Geometry: final body of the model. Coordinates: model frame, mm. Face numbers are marked on the shaded views. A direction names the side the tool comes from. Round coordinates to 2 decimals unless told otherwise and drop trailing zeros. Write each loop counter-clockwise with the first axis right and the second up, starting at its lowest first coordinate (ties: lowest second). Pieces come first, ordered by that corner, then holes. Notation, with made-up numbers: M 38.5,78 L 86.5,78 A26 ccw 86.5,92 Z; hole C 34,44.25 d6. An arc over 180 degrees is marked long. Answer as CSV lines item,"result". Start each with the question number.
Q1. Section query B-B on y = 0. Give the number of separate pieces and of enclosed holes in the cut face, and give its area (3 significant figures).
Q2. Mould query, pull axis Z, two halves, no side actions, for the marked faces 4, 5 and 6. Classes: pulls with the +Z half, pulls with the -Z half, needs draft (parallel to the pull), parting line crosses it, or undercut.
Q3. Reachability of the marked faces 1, 2 and 3 from +Z, -Z, +X, -X, +Y, -Y: full face, straight path, thin tool, end or side. Return the list, or none.
Q4. Ray query, probe 1 along Y at (x, z) = (-12.5, -1); probe 2 along Y at (x, z) = (7.5, -8.6); probe 3 along X at (y, z) = (5.25, 6.25). Return the intervals inside material, ascending.
Q5. Section query C-C on x = -17. Output: boundary loops of the cut face in (y, z).
Q6. Section query A-A on x = 7.5. Output: boundary loops of the cut face in (y, z).
Q7. First-contact query: pin 1 (2.5 mm diameter, centred on x = -12.5, y = -8.75, fed in from -Z); pin 2 (6 mm diameter, centred on x = 19, z = -2.5, fed in from +Y); pin 3 (1 mm diameter, centred on y = -8.5, z = -5.5, fed in from +X); pin 4 (1.5 mm diameter, centred on x = 23, z = -0.5, fed in from -Y). Flat tips, straight axial feed; report the tip coordinate or a pass-through.
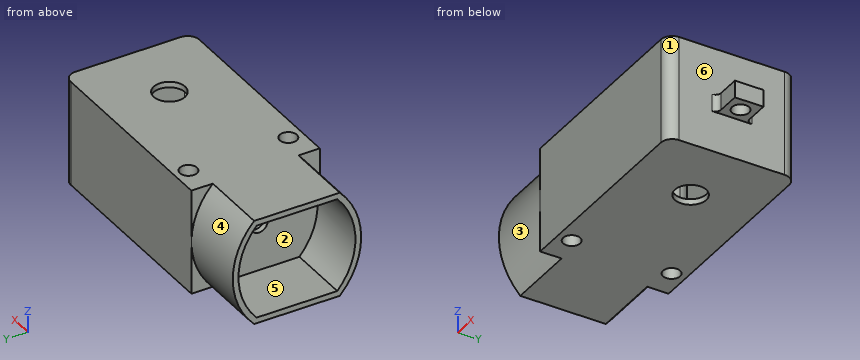
```python
from build123d import *

# Parameters (mm, degrees)
SKETCH1_R                = 1.5
BOSS_EXTRUDE1_DEPTH      = 9.22
BOSS_EXTRUDE2_DEPTH      = 12
SHELL1_START             = -10
SHELL1_OUTLINE_W         = 20.5
SHELL1_OUTLINE_H         = 16.44
SHELL1_DEPTH             = 27.5
SHELL1_START_2           = -29.5
SHELL1_2_DEPTH           = 14.5
SHELL1_START_3           = -16.5
SHELL1_3_DEPTH           = 1.5
SHELL1_START_4           = -8.22
SHELL1_4_DEPTH           = 16.44
SKETCH3_R                = 1.5
BOSS_EXTRUDE3_DEPTH      = 1
BOSS_EXTRUDE4_DEPTH      = 1.5
BOSS_EXTRUDE4_DEPTH_BACK = 1.5
SKETCH6_W                = 5
SKETCH6_H                = 5
SKETCH6_R                = 1.5
SKETCH7_R                = 2.75
CUT_EXTRUDE1_DEPTH       = 37.562906066
FILLET1_R                = 1


with BuildPart() as part:
    # Sketch1 → Boss-Extrude1 (new, symmetric)
    with BuildSketch(Plane.XY):
        with BuildLine():
            Line((17.5, -11.25), (-17.5, -11.25))
            Line((-17.5, -11.25), (-17.5, 11.25))
            Line((-17.5, 11.25), (17.5, 11.25))
            ThreePointArc((17.5, 11.25), (18.914213562, 10.664213562), (19.5, 9.25))
            Line((19.5, 9.25), (19.5, -9.25))
            ThreePointArc((19.5, -9.25), (18.914213562, -10.664213562), (17.5, -11.25))
        make_face()
        with Locations((-12.5, 8.75)):
            Circle(SKETCH1_R, mode=Mode.SUBTRACT)
        with Locations((-12.5, -8.75)):
            Circle(SKETCH1_R, mode=Mode.SUBTRACT)
    extrude(amount=BOSS_EXTRUDE1_DEPTH, both=True)

    # Sketch2 → Boss-Extrude2 (add)
    with BuildSketch(Plane.ZY.offset(17.5)):
        with BuildLine():
            Line((9.22, -7.5), (9.22, 7.5))
            ThreePointArc((9.22, 7.5), (0, 11.25), (-9.22, 7.5))
            Line((-9.22, 7.5), (-9.22, -7.5))
            ThreePointArc((-9.22, -7.5), (0, -11.25), (9.22, -7.5))
        make_face()
    extrude(amount=BOSS_EXTRUDE2_DEPTH)

    # Shell1: read off the stored shape, not the designer's step
    # Shell1 outline → Shell1 (cut)
    with BuildSketch(Plane.YZ.offset(SHELL1_START)):
        Rectangle(SHELL1_OUTLINE_W, SHELL1_OUTLINE_H)
    extrude(amount=SHELL1_DEPTH, mode=Mode.SUBTRACT)

    # Shell1 2 outline → Shell1 2 (cut)
    with BuildSketch(Plane.YZ.offset(SHELL1_START_2)):
        with BuildLine():
            ThreePointArc((7.068411902, -8.22), (10.25, 0), (7.068411902, 8.22))
            Line((7.068411902, 8.22), (-7.068411902, 8.22))
            ThreePointArc((-7.068411902, 8.22), (-10.25, 0), (-7.068411902, -8.22))
            Line((-7.068411902, -8.22), (7.068411902, -8.22))
        make_face()
    extrude(amount=SHELL1_2_DEPTH, mode=Mode.SUBTRACT)

    # Shell1 3 outline → Shell1 3 (cut)
    with BuildSketch(Plane.YZ.offset(SHELL1_START_3)):
        with BuildLine():
            Line((10.25, 0), (10.25, 8.22))
            Line((10.25, 8.22), (7.068411902, 8.22))
            ThreePointArc((7.068411902, 8.22), (9.426855331, 4.407122157), (10.25, 0))
        make_face()
        with BuildLine():
            Line((10.25, -8.22), (10.25, 0))
            ThreePointArc((10.25, 0), (9.426855331, -4.407122157), (7.068411902, -8.22))
            Line((7.068411902, -8.22), (10.25, -8.22))
        make_face()
        with BuildLine():
            ThreePointArc((-10.25, 0), (-9.426855331, 4.407122157), (-7.068411902, 8.22))
            Line((-7.068411902, 8.22), (-10.25, 8.22))
            Line((-10.25, 8.22), (-10.25, 0))
        make_face()
        with BuildLine():
            Line((-10.25, -8.22), (-7.068411902, -8.22))
            ThreePointArc((-7.068411902, -8.22), (-9.426855331, -4.407122157), (-10.25, 0))
            Line((-10.25, 0), (-10.25, -8.22))
        make_face()
    extrude(amount=SHELL1_3_DEPTH, mode=Mode.SUBTRACT)

    # Shell1 4 outline → Shell1 4 (cut)
    with BuildSketch(Plane.XY.offset(SHELL1_START_4)):
        with BuildLine():
            ThreePointArc((-14.5, -10.25), (-14.871708245, -9.540569415), (-15, -8.75))
            Line((-15, -8.75), (-15, -10.25))
            Line((-15, -10.25), (-14.5, -10.25))
        make_face()
        with BuildLine():
            ThreePointArc((-10, 8.75), (-12.499999993, 6.25), (-15, 8.749999987))
            Line((-15, 8.749999987), (-15, -8.75))
            ThreePointArc((-15, -8.75), (-12.5, -6.25), (-10, -8.75))
            Line((-10, -8.75), (-10, 8.75))
        make_face()
        with BuildLine():
            Line((-14.5, 10.25), (-15, 10.25))
            Line((-15, 10.25), (-15, 8.749999987))
            ThreePointArc((-15, 8.749999987), (-14.871708247, 9.540569409), (-14.5, 10.25))
        make_face()
        with BuildLine():
            ThreePointArc((-10.5, 10.25), (-10.128291755, 9.540569415), (-10, 8.75))
            Line((-10, 8.75), (-10, 10.25))
            Line((-10, 10.25), (-10.5, 10.25))
        make_face()
        with BuildLine():
            Line((-10, -10.25), (-10, -8.75))
            ThreePointArc((-10, -8.75), (-10.128291755, -9.540569415), (-10.5, -10.25))
            Line((-10.5, -10.25), (-10, -10.25))
        make_face()
        with BuildLine():
            ThreePointArc((18.5, 9.25), (18.207106781, 9.957106781), (17.5, 10.25))
            Line((17.5, 10.25), (17.5, -10.25))
            ThreePointArc((17.5, -10.25), (18.207106781, -9.957106781), (18.5, -9.25))
            Line((18.5, -9.25), (18.5, 9.25))
        make_face()
    extrude(amount=SHELL1_4_DEPTH, mode=Mode.SUBTRACT)

    # Sketch3 → Boss-Extrude3 (add)
    with BuildSketch(Plane.ZY.offset(17.5)):
        with BuildLine():
            Line((-9.22, 7.5), (-9.22, -7.5))
            ThreePointArc((-9.22, -7.5), (0, -11.25), (9.22, -7.5))
            Line((9.22, -7.5), (9.22, 7.5))
            ThreePointArc((9.22, 7.5), (0, 11.25), (-9.22, 7.5))
        make_face()
        Circle(SKETCH3_R, mode=Mode.SUBTRACT)
    extrude(amount=BOSS_EXTRUDE3_DEPTH)

    # Sketch6 → Boss-Extrude4 (add, two sides: drawn at the far end of the back side and taken through both)
    with BuildSketch(Plane.XY.offset(-0.58).offset(-BOSS_EXTRUDE4_DEPTH_BACK)):
        with Locations((22, 0)):
            Rectangle(SKETCH6_W, SKETCH6_H)
        with Locations((22, 0)):
            Circle(SKETCH6_R, mode=Mode.SUBTRACT)
    extrude(amount=BOSS_EXTRUDE4_DEPTH + BOSS_EXTRUDE4_DEPTH_BACK)

    # Sketch7 → Cut-Extrude1 (cut, through all)
    with BuildSketch(Plane.XY.offset(9.22)):
        with Locations((7.5, 0)):
            Circle(SKETCH7_R)
    extrude(amount=-CUT_EXTRUDE1_DEPTH, mode=Mode.SUBTRACT)

    # Fillet1
    fillet1_edges = [part.edges().sort_by_distance(p)[0] for p in [
        (19.5, 2.5, -0.58),
        (19.5, -2.5, -0.58),
    ]]
    fillet(fillet1_edges, radius=FILLET1_R)


solid = part.part
```
Entries:
1,separate pieces,"4"
1,enclosed holes,"0"
1,area,"123 mm^2"
2,face 4,"parting line crosses it"
2,face 5,"undercut"
2,face 6,"needs draft"
3,face 1,"+Z, -Z, +X, -Y"
3,face 2,"-X"
3,face 3,"-X, -Y"
4,probe 1,"y = -11.25 to -10.25, -7.25 to -6.25, 6.25 to 7.25, 10.25 to 11.25"
4,probe 2,"y = -11.25 to -2.75, 2.75 to 11.25"
4,probe 3,"x = -18.5 to -17.5, 18.5 to 19.5"
5,outline,"M -11.25,-9.22 L 11.25,-9.22 L 11.25,9.22 L -11.25,9.22 Z; hole M -7.07,-8.22 L 7.07,-8.22 A12.21 ccw 7.07,8.22 L -7.07,8.22 A12.21 ccw Z"
6,outline,"M -11.25,-9.22 L -2.75,-9.22 L -2.75,-8.22 L -10.25,-8.22 L -10.25,8.22 L -2.75,8.22 L -2.75,9.22 L -11.25,9.22 Z; M 2.75,-9.22 L 11.25,-9.22 L 11.25,9.22 L 2.75,9.22 L 2.75,8.22 L 10.25,8.22 L 10.25,-8.22 L 2.75,-8.22 Z"
7,pin 1,"passes through"
7,pin 2,"stops at y = 11.25"
7,pin 3,"stops at x = 19.5"
7,pin 4,"stops at y = -2.5"
